The model under review builds one solid part; all positions refer to its coordinate system, in mm. Face numbers are marked on the shaded views. A direction names the side the tool comes from. Coordinates: 2 decimals unless noted, no trailing zeros. Write each loop counter-clockwise with the first axis right and the second up, starting at its lowest first coordinate (ties: lowest second). Pieces come first, ordered by that corner, then holes. Notation, with made-up numbers: (77.25, 24.5) - (100.25, 24.5) arc R17 ccw to (100.25, 28.5) - close; hole circle Ø10 at (42, 15.25). An arc over 180 degrees is marked (long way). Return JSON: item names as keys, results as strings. Group by question number.
(1) To check wall thickness, follow L1, parallel to Y at x = 25, z = 0; L2, parallel to Y at x = 11, z = 0; L3, parallel to X at y = 7, z = 4.25. State the ranges of each line that lie inside material, in increasing order. Write a range as from..to.
(2) Tool access review of the marked faces 4, 5 and 6: name each direction out of +Z, -Z, +X, -X, +Y, -Y from which nothing blocks a thin tool from reaching the whole face with its end or side.
(3) We need section C-C on x = 13.5. State the section outline as (y, z) points, then the cut area to 3 significant figures.
(4) We need section D-D on x = 21. State the section outline as (y, z) points.
(5) We need section A-A on y = 0. State the section outline as (x, z) points.
(6) Draft analysis for pull direction X (two halves, no side actions). For the marked faces 1, 2 and 3, state which applies: released by +X, released by -X, zero draft, split by the parting line, or undercut.
(7) For pin 1 Ø3 at (x, z) = (21, 0.5) entering from -Y; pin 2 Ø6 at (x, z) = (29, 4) entering from +Y; pin 3 Ø1 at (x, y) = (23.5, -4) entering from -Z, all flat-tipped, find the tip position at first contact; note any pin that passes through.
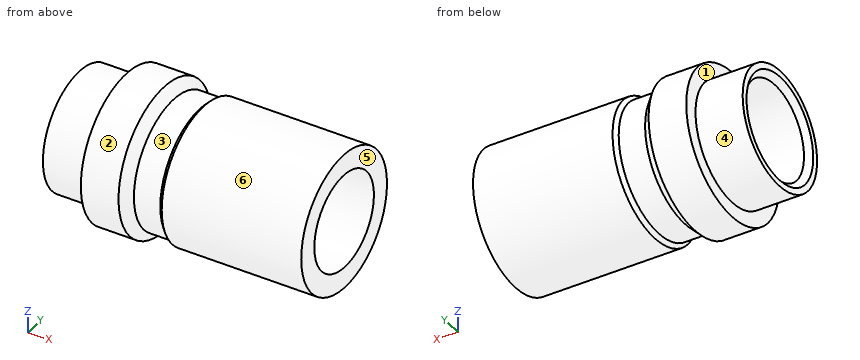
```python
from build123d import *

# Parameters (mm, degrees)
F_1_2_0_5_DIAMETER_HOLE1_D = 12.7
CHAMFER1_SIZE              = 0.762


with BuildPart() as part:
    # Sketch1 → Revolve1 (revolve)
    with BuildSketch(Plane.XY):
        Polygon((6.35, 7.9375), (6.35, 9.906), (11.43, 9.906), (12.7, 8.636), (16.256, 8.636), (16.764, 9.144), (35.56, 9.144), (35.56, 5.08), (35.56, 0), (0, 0), (0, 7.9375), align=None)
    revolve(axis=Axis((35.56, 0, 0), (-1, 0, 0)))

    # 1/2 (0.5) Diameter Hole1 (through all)
    with Locations(Plane.ZY):
        with Locations((0, 0)):
            Hole(F_1_2_0_5_DIAMETER_HOLE1_D / 2)

    # Chamfer1
    chamfer1_edges = [part.edges().sort_by_distance(p)[0] for p in [
        (0, 0, 6.35),
    ]]
    chamfer(chamfer1_edges, length=CHAMFER1_SIZE)


solid = part.part
```
Ans:
{
 "1": {"L1": "-9.14..-6.35, 6.35..9.14", "L2": "-9.91..-6.35, 6.35..9.91", "L3": "6.35..35.56"},
 "2": {"face 4": "-X", "face 5": "+Z, -Z, +X, +Y, -Y", "face 6": "+X"},
 "3": {"outline": "circle Ø17.27 at (0, 0); hole circle Ø12.7 at (0, 0)", "area": "108 mm²"},
 "4": {"outline": "circle Ø18.29 at (0, 0); hole circle Ø12.7 at (0, 0)"},
 "5": {"outline": "(0, -7.94) - (6.35, -7.94) - (6.35, -9.91) - (11.43, -9.91) - (12.7, -8.64) - (16.26, -8.64) - (16.76, -9.14) - (35.56, -9.14) - (35.56, -6.35) - (0.76, -6.35) - (0, -7.11) - close; (0, 7.11) - (0.76, 6.35) - (35.56, 6.35) - (35.56, 9.14) - (16.76, 9.14) - (16.26, 8.64) - (12.7, 8.64) - (11.43, 9.91) - (6.35, 9.91) - (6.35, 7.94) - (0, 7.94) - close"},
 "6": {"face 1": "released by -X", "face 2": "zero draft", "face 3": "undercut"},
 "7": {"pin 1": "y = -9.14", "pin 2": "y = 9.09", "pin 3": "z = -8.45"}
}
